The listing builds one solid part. Answer for the finished solid, in the listing's coordinates (mm). Face numbers are marked on the shaded views. A direction names the side the tool comes from. Coordinates: 2 decimals unless noted, no trailing zeros. Write each loop counter-clockwise with the first axis right and the second up, starting at its lowest first coordinate (ties: lowest second). Pieces come first, ordered by that corner, then holes.
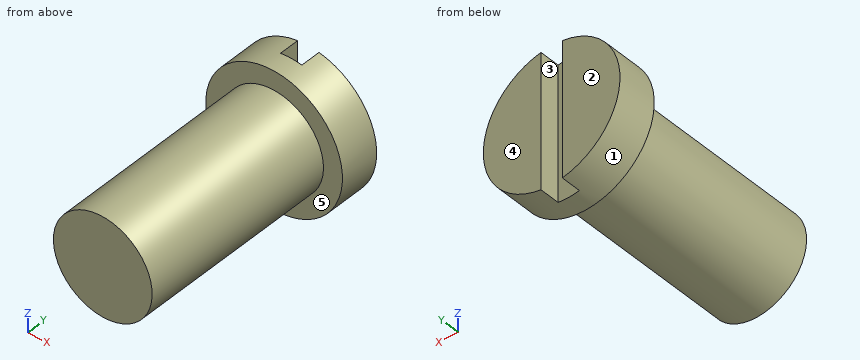
from build123d import *

# Parameters (mm, degrees)
CUT_EXTRUDE1_REACH                  = 14.959
CUT_EXTRUDE1_END_RADIUS             = 3.46
SKETCH2_W                           = 1.08
SKETCH2_H                           = 1
CUT_EXTRUDE1_DIRECTION_2_REACH      = 14.959
CUT_EXTRUDE1_DIRECTION_2_END_RADIUS = 3.46


with BuildPart() as part:
    # Sketch1 → Revolve1 (revolve)
    with BuildSketch(Plane.XY, mode=Mode.PRIVATE) as revolve1_sk:
        Polygon((0, 12), (3.46, 12), (3.46, 10), (2.5, 10), (2.5, 0), (0, 0), align=None)
    revolve(revolve1_sk.sketch.rotate(Axis((0, 0, 0), (0, 1, 0)), 90), axis=Axis((0, 0, 0), (0, 1, 0)))

    # Cut-Extrude1: up to this cylinder (the profile starts inside it)
    cut_extrude1_end = Plane(origin=(0, 11.5, 0), z_dir=(0, -1, 0)) * Cylinder(CUT_EXTRUDE1_END_RADIUS, 37.838, mode=Mode.PRIVATE)
    # Sketch2 → Cut-Extrude1 (cut, up to the surface)
    with BuildSketch(Plane.XY, mode=Mode.PRIVATE) as cut_extrude1_sk1:
        with Locations((0, 11.5)):
            Rectangle(SKETCH2_W, SKETCH2_H)
    cut_extrude1_tool1 = extrude(cut_extrude1_sk1.sketch, amount=-CUT_EXTRUDE1_REACH, mode=Mode.PRIVATE) & cut_extrude1_end
    add(cut_extrude1_tool1.solids().sort_by_distance((0, 11.5, 0))[0], mode=Mode.SUBTRACT)

    # Cut-Extrude1 direction 2: up to this cylinder (the profile starts inside it)
    cut_extrude1_direction_2_end = Plane(origin=(0, 11.5, 0), z_dir=(0, -1, 0)) * Cylinder(CUT_EXTRUDE1_DIRECTION_2_END_RADIUS, 37.838, mode=Mode.PRIVATE)
    # Sketch2 → Cut-Extrude1 direction 2 (cut, up to the surface)
    with BuildSketch(Plane.XY, mode=Mode.PRIVATE) as cut_extrude1_direction_2_sk1:
        with Locations((0, 11.5)):
            Rectangle(SKETCH2_W, SKETCH2_H)
    cut_extrude1_direction_2_tool1 = extrude(cut_extrude1_direction_2_sk1.sketch, amount=CUT_EXTRUDE1_DIRECTION_2_REACH, mode=Mode.PRIVATE) & cut_extrude1_direction_2_end
    add(cut_extrude1_direction_2_tool1.solids().sort_by_distance((0, 11.5, 0))[0], mode=Mode.SUBTRACT)


solid = part.part
Q1. The part is cut by section B-B, the plane x = 0. Write down the section's boundary in (y, z), then the cut area to 3 significant figures.
Answers below:
outline: (0, -2.5) - (10, -2.5) - (10, -3.46) - (11, -3.46) - (11, 3.46) - (10, 3.46) - (10, 2.5) - (0, 2.5) - close
area: 56.9 mm2
Q2. Determine the mould class of the marked faces 1, 2 and 3 for opening direction X: released by +X, released by -X, zero draft, split by the parting line, or undercut.
Answers below:
face 1: split by the parting line
face 2: zero draft
face 3: undercut
Q3. Given pin 1 (0.5 mm diameter, centred on y = 11.5, z = 1, fed in from -X); pin 2 (3 mm diameter, centred on y = 2, z = 0, fed in from +X); pin 3 (0.8 mm diameter, centred on y = 11.5, z = 1, fed in from +X); pin 4 (3.5 mm diameter, centred on x = 0, z = 0.5, fed in from -Y), each flat-ended and moving along its own axis, determine where each tip first touches the part or whether it passes through.
Answers below:
pin 1: stops at x = -3.38
pin 2: stops at x = 2.5
pin 3: stops at x = 3.41
pin 4: stops at y = 0
Q4. The part is cut by section A-A, the plane z = 0. Write down the section's boundary in (x, y).
Answers below:
outline: (-3.46, 10) - (-2.5, 10) - (-2.5, 0) - (2.5, 0) - (2.5, 10) - (3.46, 10) - (3.46, 12) - (0.54, 12) - (0.54, 11) - (-0.54, 11) - (-0.54, 12) - (-3.46, 12) - close
Q5. Which of the six approach directions +Z, -Z, +X, -X, +Y, -Y give full straight-line access (tool end or side, diameter ignored) to the marked faces 4 and 5?
Answers below:
face 4: +Z, -Z, +X, -X, +Y
face 5: -Y
Q6. The part is cut by section C-C, the plane y = 1.75. Write down the section's boundary in (x, z), then the cut area to 3 significant figures.
Answers below:
outline: circle Ø5 at (0, 0)
area: 19.6 mm2
Q7. The part is cut by section D-D, the plane x = -1.75. Write down the section's boundary in (y, z).
Answers below:
outline: (0, -1.79) - (10, -1.79) - (10, -2.98) - (12, -2.98) - (12, 2.98) - (10, 2.98) - (10, 1.79) - (0, 1.79) - close
Q8. Find the intervals of material crossed by probe 1 along Y at (x, z) = (2.75, -1.75); probe 2 along Y at (x, z) = (0.5, 0); probe 3 along X at (y, z) = (1.75, 1.5), in increasing order.
Answers below:
probe 1: y = 10 to 12
probe 2: y = 0 to 11
probe 3: x = -2 to 2
